Check sheet for the modelled part. Datum: model origin and axes. Units: mm. A direction names the side the tool comes from. Round coordinates to 2 decimals unless told otherwise and drop trailing zeros. Order: outer loops, then holes, each group sorted by start corner. A loop starts at its lowest first (then second) coordinate and runs counter-clockwise, first axis right, second up. Notation, with made-up numbers: (7.25, 46.25) -> (26.25, 46.25) arc R20 cw to (26.25, 84.25) -> close; hole circle Ø5 at (-28, 67.5). An arc over 180 degrees is marked (long way). Answer in a Markdown table with one row per item.
```python
from build123d import *

# Parameters (mm, degrees)
F0_R           = 55
F0_R_2         = 30
F0_R_3         = 21
F0_R_4         = 12.5
F1_DEPTH       = 20
F2_DEPTH       = 1.6
F3_R           = 30
F3_R_2         = 12.5
F4_DEPTH       = 4
F5_D           = 5
F5_DEPTH       = 12
F5_CBORE_D     = 6
F5_CBORE_DEPTH = 1
F5_TIP         = 1.5021515476
F6_D           = 13
F6_CBORE_D     = 20
F6_CBORE_DEPTH = 10
F7_D           = 6.8
F7_CBORE_D     = 8
F7_CBORE_DEPTH = 1.2
F8_SIZE2       = 0.5
F8_SIZE        = 0.5
F9_R           = 0.3


with BuildPart() as f1:
    # F0 (on Right) → F1 (new body)
    with BuildSketch(Plane.YZ):
        Circle(F0_R)
        Circle(F0_R_2, mode=Mode.SUBTRACT)
        Circle(F0_R_2)
        Circle(F0_R_3, mode=Mode.SUBTRACT)
        Circle(F0_R_3)
        Circle(F0_R_4, mode=Mode.SUBTRACT)
    extrude(amount=F1_DEPTH)

    # F0 (on Right) → F2 (join)
    with BuildSketch(Plane.YZ):
        Circle(F0_R_3)
        Circle(F0_R_4, mode=Mode.SUBTRACT)
    extrude(amount=-F2_DEPTH)

    # F3 (on face) → F4 (join)
    with BuildSketch(Plane.YZ.offset(20)):
        Circle(F3_R)
        Circle(F3_R_2, mode=Mode.SUBTRACT)
    extrude(amount=F4_DEPTH)

    # F5
    with Locations(Plane(origin=(0, 0, 0), x_dir=(0, 1, 0), z_dir=(-1, 0, 0))):
        with Locations((-15.5, -26.8467875173), (-31, 0), (-15.5, 26.8467875173), (15.5, -26.8467875173), (31, 0), (15.5, 26.8467875173)):
            CounterBoreHole(F5_D / 2, F5_CBORE_D / 2, F5_CBORE_DEPTH, depth=F5_DEPTH)
            with Locations((0, 0, -(F5_DEPTH + F5_TIP / 2))):  # 118° drill point
                Cone(0, F5_D / 2, F5_TIP, mode=Mode.SUBTRACT)

    # F6 (through all)
    with Locations(Plane(origin=(0, 0, 0), x_dir=(0, 1, 0), z_dir=(-1, 0, 0))):
        with Locations((-32.8214868646, 27), (-32.8214868646, -27), (32.8214868646, -27), (32.8214868646, 27)):
            CounterBoreHole(F6_D / 2, F6_CBORE_D / 2, F6_CBORE_DEPTH)

    # F7 (through all)
    with Locations(Plane(origin=(0, 0, 0), x_dir=(0, 1, 0), z_dir=(-1, 0, 0))):
        with Locations((0, -42.5), (0, 42.5)):
            CounterBoreHole(F7_D / 2, F7_CBORE_D / 2, F7_CBORE_DEPTH)

    # F8
    f8_edges = [f1.edges().sort_by_distance(p)[0] for p in [
        (20, -55, 0),
        (0, -55, 0),
        (24, -30, 0),
        (24, -12.5, 0),
        (-1.6, -12.5, 0),
    ]]
    chamfer(f8_edges, length=F8_SIZE, length2=F8_SIZE2)

    # F9
    f9_edges = [f1.edges().sort_by_distance(p)[0] for p in [
        (20, -30, 0),
        (0, -21, 0),
        (-1.6, -21, 0),
    ]]
    fillet(f9_edges, radius=F9_R)


solid = f1.part
```
(1) Draft check along Y on faces 3 (the cylindrical face through (6.58, 17.34, -28.54)), 4 (the cylindrical face through (-0.79, 20.03, 6.31)). Enter one of: pulls with the +Y half, pulls with the -Y half, needs draft (parallel to the pull), parting line crosses it, or undercut.
Solutions:
| item | result |
|---|---|
| face 3 | undercut |
| face 4 | parting line crosses it |
(2) Section check A-A on x = 16.5. Record the boundary of the cut face in (y, z), plus the area to 3 significant figures.
Solutions:
| item | result |
|---|---|
| outline | circle Ø110 at (0, 0); hole circle Ø13 at (-32.82, -27); hole circle Ø13 at (-32.82, 27); hole circle Ø25 at (0, 0); hole circle Ø6.8 at (0, -42.5); hole circle Ø6.8 at (0, 42.5); hole circle Ø13 at (32.82, -27); hole circle Ø13 at (32.82, 27) |
| area | 8,410 mm^2 |
(3) Section check B-B on y = 0. Give the number of separate pieces and of enclosed holes in the cut face, plus the area to 3 significant figures.
Solutions:
| item | result |
|---|---|
| separate pieces | 4 |
| enclosed holes | 0 |
| area | 1,590 mm^2 |
(4) Depth check by flat-ended pin: pin 1 Ø8 at (y, z) = (-22, -41.5) entering from +X; pin 2 Ø10 at (x, y) = (15.5, 3) entering from -Z; pin 3 Ø2 at (y, z) = (-32, 13.5) entering from -X. Enter the tip coordinate at first touch or a pass-through.
Solutions:
| item | result |
|---|---|
| pin 1 | x = 20 |
| pin 2 | z = -55 |
| pin 3 | x = 0 |
(5) Tool access check on faces 1 (the cylindrical face through (9.867, -11.923, -53.692)), 2 (the cylindrical face through (0.592, -0.521, 38.534)). Record the directions out of +Z, -Z, +X, -X, +Y, -Y that give a thin tool (end or side, any length) a straight path to the whole face; none if there is none.
Solutions:
| item | result |
|---|---|
| face 1 | +X, -X |
| face 2 | -X |
(6) Scan lines: probe 1 along Z at (x, y) = (0.5, 0); probe 2 along Y at (x, z) = (12.25, 27); probe 3 along Y at (x, z) = (12.5, -27). Record each from-to range of solid material in increasing order. Write a range as from..to.
Solutions:
| item | result |
|---|---|
| probe 1 | -55..-46.5, -38.5..-12.5, 12.5..38.5, 46.5..55 |
| probe 2 | -47.92..-39.32, -26.32..-17.58, -13.42..13.42, 17.58..26.32, 39.32..47.92 |
| probe 3 | -47.92..-39.32, -26.32..-17.16, -13.84..13.84, 17.16..26.32, 39.32..47.92 |
